Read the model definition and answer for the solid it produces. Units are mm, in the model's axes. A direction names the side the tool comes from. Coordinates: 2 decimals unless noted, no trailing zeros. Write each loop counter-clockwise with the first axis right and the second up, starting at its lowest first coordinate (ties: lowest second). Pieces come first, ordered by that corner, then holes. Notation, with made-up numbers: (-29.5, 24.25) -> (-10.5, 24.25) arc R21 ccw to (-10.5, 36.25) -> close; hole circle Ø10 at (-13.75, -22.75). An arc over 180 degrees is marked (long way). Return JSON: item names as keys, results as strings.
from build123d import *

# Parameters (mm, degrees)
SKETCH_1_R      = 11
SKETCH_1_R_2    = 3.5
SKETCH_1_R_3    = 1.01
SKETCH_1_R_4    = 6
SKETCH_1_R_5    = 4.025
EXTRUDE_1_DEPTH = 3
SKETCH_2_R      = 1.525
EXTRUDE_2_DEPTH = 3
FILLET_1_R      = 2


with BuildPart() as part:
    # 草图1 → 凸台-拉伸1 (new body)
    # profile 1 of 3: a face of its own
    with BuildSketch(Plane.XY):
        with BuildLine():
            ThreePointArc((10.983011573, -0.611111111), (0, -11), (-10.983011573, -0.611111111))
            Line((-10.983011573, -0.611111111), (-5.990733585, -90.333333333))
            ThreePointArc((-5.990733585, -90.333333333), (-0.166731054, -84.002317051), (6, -90))
            ThreePointArc((6, -90), (5.997682949, -90.166731054), (5.990733585, -90.333333333))
            Line((5.990733585, -90.333333333), (10.983011573, -0.611111111))
        make_face()
        with BuildLine():
            Line((-3.466771313, -81.694489982), (-7.418369738, -10.675569794))
            ThreePointArc((-7.418369738, -10.675569794), (0, -13), (7.418369738, -10.675569794))
            Line((7.418369738, -10.675569794), (3.466771313, -81.694489982))
            ThreePointArc((3.466771313, -81.694489982), (0, -81), (-3.466771313, -81.694489982))
        make_face(mode=Mode.SUBTRACT)
    # profile 2 of 3: a face of its own
    with BuildSketch(Plane.XY):
        Circle(SKETCH_1_R)
        Circle(SKETCH_1_R_2, mode=Mode.SUBTRACT)
        with Locations((-2.75, 4.763139721)):
            Circle(SKETCH_1_R_3, mode=Mode.SUBTRACT)
        with Locations((-2.75, -4.763139721)):
            Circle(SKETCH_1_R_3, mode=Mode.SUBTRACT)
        with Locations((5.5, 0)):
            Circle(SKETCH_1_R_3, mode=Mode.SUBTRACT)
    # profile 3 of 3: a face of its own
    with BuildSketch(Plane.XY):
        with Locations((0, -90)):
            Circle(SKETCH_1_R_4)
        with Locations((0, -90)):
            Circle(SKETCH_1_R_5, mode=Mode.SUBTRACT)
    extrude(amount=EXTRUDE_1_DEPTH)

    # 草图2 → 凸台-拉伸2 (add)
    with BuildSketch(Plane.XY.offset(3)):
        Polygon((-6.745155967, -22.774702841), (6.745155967, -22.774702841), (6.411307036, -28.774702841), (-6.411307036, -28.774702841), align=None)
        with Locations((-4.5, -25.774702841)):
            Circle(SKETCH_2_R, mode=Mode.SUBTRACT)
        with Locations((4.5, -25.774702841)):
            Circle(SKETCH_2_R, mode=Mode.SUBTRACT)
    extrude(amount=-EXTRUDE_2_DEPTH)

    # 圆角1
    fillet_1_edges = [part.edges().sort_by_distance(p)[0] for p in [
        (7.418369738, -10.675569794, 1.5),
        (-7.418369738, -10.675569794, 1.5),
        (-3.466771313, -81.694489982, 1.5),
        (3.466771313, -81.694489982, 1.5),
        (6.411307036, -28.774702841, 1.5),
        (6.745155967, -22.774702841, 1.5),
        (-6.745155967, -22.774702841, 1.5),
        (-6.411307036, -28.774702841, 1.5),
    ]]
    fillet(fillet_1_edges, radius=FILLET_1_R)


solid = part.part
1. The part is cut by section B-B (y = -60). Determine the outline of the cut face in (x, z).
Taken from the geometry:
{"outline": "(-7.68, 0) -> (-4.67, 0) -> (-4.67, 3) -> (-7.68, 3) -> close; (4.67, 0) -> (7.68, 0) -> (7.68, 3) -> (4.67, 3) -> close"}
2. The part is cut by section C-C (z = 1.4). Count the separate pieces of the cut face and the enclosed holes in it, then the cut area to 3 significant figures.
Taken from the geometry:
{"separate pieces": "1", "enclosed holes": "9", "area": "1,010 mm2"}
3. The part is cut by section D-D (y = -82). Determine the outline of the cut face in (x, z), then the cut area to 3 significant figures.
Taken from the geometry:
{"outline": "(-6.45, 0) -> (6.45, 0) -> (6.45, 3) -> (-6.45, 3) -> close", "area": "38.7 mm2"}
4. A tool of negligible diameter and unlimited length cuts with its end or side. For faces 1 (the face through (8.45, -46.1, 1.48)), 2 (the face through (6.391, -12.434, 1.521)), from which of +Z, -Z, +X, -X, +Y, -Y can it reach the whole face along a straight path? Write none if from no direction.
Taken from the geometry:
{"face 1": "+Z, -Z, +X, -Y", "face 2": "+Z, -Z"}
5. Consider L1, parallel to X at y = -25, z = 0.7; L2, parallel to X at y = -39, z = 1.25; L3, parallel to X at y = -38, z = 2.35. Determine where each line is inside the solid, lowest interval first.
Taken from the geometry:
{"L1": "x = -9.63 to -5.81, -3.19 to 3.19, 5.81 to 9.63", "L2": "x = -8.85 to -5.84, 5.84 to 8.85", "L3": "x = -8.9 to -5.9, 5.9 to 8.9"}
6. For a pull along X with two mould halves and no side action, classify faces 3 (the face through (7, -30, 3)), 4 (the face through (2.89, -80.65, 1.52)), 5 (the face through (0, -96, 1)) as +X half, -X half, draft (parallel to the pull), parting line (faces both ways), or undercut.
Taken from the geometry:
{"face 3": "draft", "face 4": "undercut", "face 5": "parting line"}
7. Flat-ended cylindrical pins translate along their axes: pin 1 Ø1 at (y, z) = (-83, 0.5) entering from -X; pin 2 Ø0.9 at (x, z) = (1.5, 2) entering from +Y. Find the tip coordinate at first contact, or state that the pin passes through.
Taken from the geometry:
{"pin 1": "stops at x = -6.43", "pin 2": "stops at y = 10.95"}
8. The part is cut by section A-A (x = 0). Determine the outline of the cut face in (y, z) (3 decimals).
Taken from the geometry:
{"outline": "(-96, 0) -> (-94.025, 0) -> (-94.025, 3) -> (-96, 3) -> close; (-85.975, 0) -> (-81, 0) -> (-81, 3) -> (-85.975, 3) -> close; (-28.775, 0) -> (-22.775, 0) -> (-22.775, 3) -> (-28.775, 3) -> close; (-13, 0) -> (-3.5, 0) -> (-3.5, 3) -> (-13, 3) -> close; (3.5, 0) -> (11, 0) -> (11, 3) -> (3.5, 3) -> close"}
